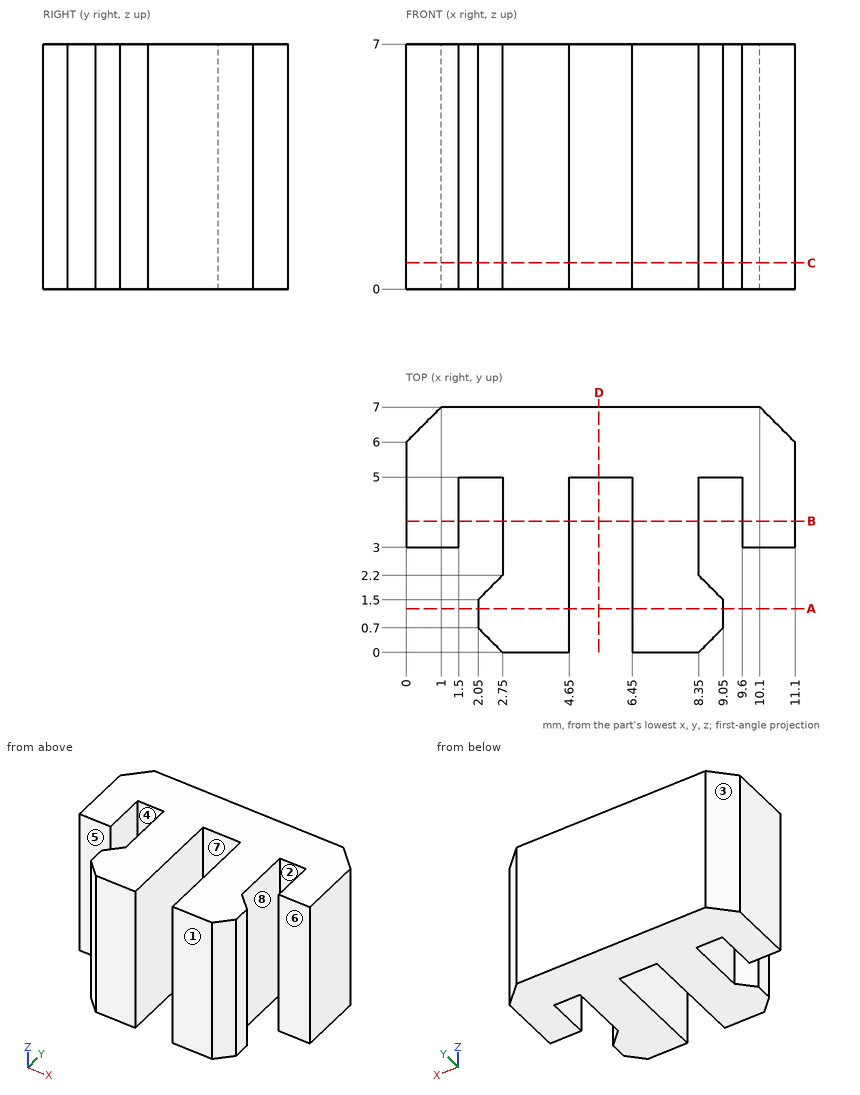
Answer from the drawing. Dimensions are ordinates in mm from the lowest x, y and z of the part. A direction names the side the tool comes from. Give positions to 0.01 mm unless a question says otherwise; leave off trailing zeros. Write each loop counter-clockwise with the first axis right and the second up, starting at its lowest first coordinate (ties: lowest second). Pieces come first, ordered by that corner, then holes. Notation, with made-up numbers: (81, 53) -> (88, 53) arc R23 ccw to (88, 63) -> close; hole circle Ø6 at (-32.5, -34). An arc over 180 degrees is marked (long way). One line per question, with ' | ' between items. Start each with the question number.
1. Section B-B (y = 3.75) is taken. Determine the outline of the cut face in (x, z), plus the area to 3 significant figures.
2. Section C-C (z = 0.75) is taken. Determine the outline of the cut face in (x, y), plus the area to 3 significant figures.
3. Find the intervals of material crossed by probe 1 along X at (y, z) = (4.25, 3.5); probe 2 along X at (y, z) = (1, 1.75); probe 3 along Y at (x, z) = (4.75, 2), in increasing order.
4. Given pin 1 Ø1.2 at (x, z) = (1, 2) entering from -Y; pin 2 Ø1 at (x, z) = (2, 4.5) entering from -Y; pin 3 Ø1 at (y, z) = (1, 4) entering from +X, each flat-ended and moving along its own axis, determine where each tip first touches the part or whether it passes through.
5. Section A-A (y = 1.25) is taken. Determine the outline of the cut face in (x, z), plus the area to 3 significant figures.
6. For the marked faces 5, 6, 7 and 8, determine the directions among +Z, -Z, +X, -X, +Y, -Y from which every point of the face is accessible in a straight line to the end or side of a thin tool.
7. For a pull along Y with two mould halves and no side action, classify the marked faces 1, 2, 3 and 4 as pulls with the +Y half, pulls with the -Y half, needs draft (parallel to the pull), parting line crosses it, or undercut.
8. Section D-D (x = 5.5) is taken. Determine the outline of the cut face in (y, z), plus the area to 3 significant figures.
Response values:
1) outline: (0, 0) -> (1.5, 0) -> (1.5, 7) -> (0, 7) -> close; (2.75, 0) -> (4.65, 0) -> (4.65, 7) -> (2.75, 7) -> close; (6.45, 0) -> (8.35, 0) -> (8.35, 7) -> (6.45, 7) -> close; (9.6, 0) -> (11.1, 0) -> (11.1, 7) -> (9.6, 7) -> close | area: 47.6 mm2
2) outline: (0, 3) -> (1.5, 3) -> (1.5, 5) -> (2.75, 5) -> (2.75, 2.2) -> (2.05, 1.5) -> (2.05, 0.7) -> (2.75, 0) -> (4.65, 0) -> (4.65, 5) -> (6.45, 5) -> (6.45, 0) -> (8.35, 0) -> (9.05, 0.7) -> (9.05, 1.5) -> (8.35, 2.2) -> (8.35, 5) -> (9.6, 5) -> (9.6, 3) -> (11.1, 3) -> (11.1, 6) -> (10.1, 7) -> (1, 7) -> (0, 6) -> close | area: 48.3 mm2
3) probe 1: 0 to 1.5, 2.75 to 4.65, 6.45 to 8.35, 9.6 to 11.1 | probe 2: 2.05 to 4.65, 6.45 to 9.05 | probe 3: 5 to 7
4) pin 1: y = 3 | pin 2: y = 0.25 | pin 3: x = 9.05
5) outline: (2.05, 0) -> (4.65, 0) -> (4.65, 7) -> (2.05, 7) -> close; (6.45, 0) -> (9.05, 0) -> (9.05, 7) -> (6.45, 7) -> close | area: 36.4 mm2
6) face 5: +Z, -Z, -X, -Y | face 6: +Z, -Z, +X, -Y | face 7: +Z, -Z, -Y | face 8: +Z, -Z
7) face 1: pulls with the -Y half | face 2: undercut | face 3: pulls with the +Y half | face 4: undercut
8) outline: (5, 0) -> (7, 0) -> (7, 7) -> (5, 7) -> close | area: 14.0 mm2
